from build123d import *

# Parameters (mm, degrees)
SKETCH1_W           = 80
SKETCH1_H           = 14
BOSS_EXTRUDE1_DEPTH = 2
SKETCH2_W           = 80
SKETCH2_H           = 7.4
SKETCH2_H_2         = 4.9
BOSS_EXTRUDE2_DEPTH = 2
SKETCH3_W           = 28.7
SKETCH3_H           = 7
BOSS_EXTRUDE3_DEPTH = 4
BOSS_EXTRUDE4_DEPTH = 80
CUT_EXTRUDE1_DEPTH  = 1
BOSS_EXTRUDE5_DEPTH = 1.8
SKETCH7_W           = 47.6
SKETCH7_H           = 7.55
CUT_EXTRUDE2_DEPTH  = 1


with BuildPart() as part:
    # Sketch1 → Boss-Extrude1 (new body)
    with BuildSketch(Plane(origin=(0, 0, 0), x_dir=(1, 0, 0), z_dir=(0, 1, 0))):
        with Locations((32.454545455, 2.136363636)):
            Rectangle(SKETCH1_W, SKETCH1_H)
    extrude(amount=BOSS_EXTRUDE1_DEPTH)

    # Sketch2 → Boss-Extrude2 (add)
    with BuildSketch(Plane(origin=(0, 2, 0), x_dir=(1, 0, 0), z_dir=(0, 1, 0))):
        with Locations((32.454545455, -1.163636364)):
            Rectangle(SKETCH2_W, SKETCH2_H)
        with Locations((32.454545455, 6.686363636)):
            Rectangle(SKETCH2_W, SKETCH2_H_2)
    extrude(amount=BOSS_EXTRUDE2_DEPTH)

    # Sketch3 → Boss-Extrude3 (add)
    with BuildSketch(Plane.XZ):
        with Locations((6.804545455, -12.636363636)):
            Rectangle(SKETCH3_W, SKETCH3_H)
    extrude(amount=-BOSS_EXTRUDE3_DEPTH)

    # Sketch4 → Boss-Extrude4 (add)
    with BuildSketch(Plane.ZY.offset(7.545454545)):
        Polygon((-2.536363636, 2), (-2.686363636, 4), (-2.536363636, 4), align=None)
        Polygon((-4.236363636, 2), (-4.236363636, 4), (-4.086363636, 4), align=None)
    extrude(amount=-BOSS_EXTRUDE4_DEPTH)

    # Sketch5 → Cut-Extrude1 (cut)
    with BuildSketch(Plane.XZ):
        Polygon((-7.545454545, 4.863636364), (72.454545455, 4.863636364), (72.454545455, -9.136363636), (21.154545455, -9.136363636), (21.154545455, -16.136363636), (-7.545454545, -16.136363636), align=None)
    extrude(amount=-CUT_EXTRUDE1_DEPTH, mode=Mode.SUBTRACT)

    # Sketch6 → Boss-Extrude5 (add)
    with BuildSketch(Plane.XZ.offset(-1)):
        Polygon((21.154545455, -9.136363636), (72.454545455, -9.136363636), (72.454545455, -11.136363636), (23.154545455, -11.136363636), (23.154545455, -16.136363636), (21.154545455, -16.136363636), (21.154545455, -11.136363636), align=None)
    extrude(amount=-BOSS_EXTRUDE5_DEPTH)

    # Sketch7 → Cut-Extrude2 (cut)
    with BuildSketch(Plane(origin=(0, 4, 0), x_dir=(1, 0, 0), z_dir=(0, 1, 0))):
        with Locations((45.254545455, -1.088636364)):
            Rectangle(SKETCH7_W, SKETCH7_H)
    extrude(amount=-CUT_EXTRUDE2_DEPTH, mode=Mode.SUBTRACT)


solid = part.part
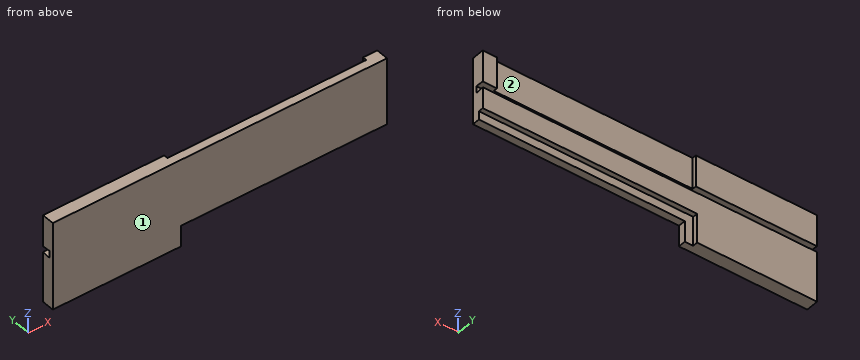
Source: CAD feature listing. Evaluate the final solid. Frame: model axes, mm. Face numbers are marked on the shaded views. Round coordinates to 2 decimals unless told otherwise and drop trailing zeros. Loops run counter-clockwise (first coordinate to the right, second up) from the corner with the lowest first, then second, coordinate; pieces in that order, holes last. Notation, with made-up numbers: M 7.25,36 L 32.25,36 A24 ccw 32.25,70 Z; hole C 89,-13 d11. An arc over 180 degrees is marked long. Answer as CSV lines item,"result".
Q1. Contact query for flat-ended pins moving along their axis: pin 1 (0.6 mm diameter, centred on x = 45, y = 3.5, fed in from -Z); pin 2 (3.5 mm diameter, centred on x = 42.5, z = 1, fed in from +Y); pin 3 (0.9 mm diameter, centred on x = 59, y = 1.5, fed in from -Z). Output: stop coordinate, or through.
Verdict:
pin 1,"stops at z = -9.14"
pin 2,"stops at y = 3"
pin 3,"stops at z = -11.14"
Q2. Cut plane A-A (x = 61). Return the cut outline in (y, z), plus the area to 3 significant figures.
Verdict:
outline,"M 1,-11.14 L 2.8,-11.14 L 2.8,-9.14 L 4,-9.14 L 4,-4.09 L 2,-4.24 L 2,-2.54 L 3,-2.61 L 3,4.86 L 1,4.86 Z"
area,"35.0 mm^2"
Q3. Cut plane D-D (x = 12.5). Return the cut outline in (y, z), plus the area to 3 significant figures.
Verdict:
outline,"M 1,-16.14 L 4,-16.14 L 4,-4.09 L 2,-4.24 L 2,-2.54 L 4,-2.69 L 4,4.86 L 1,4.86 Z"
area,"59.9 mm^2"
Q4. Cut plane C-C (z = -1.25). Return the cut outline in (x, y), plus the area to 3 significant figures.
Verdict:
outline,"M -7.55,1 L 72.45,1 L 72.45,4 L 69.05,4 L 69.05,3 L 21.45,3 L 21.45,4 L -7.55,4 Z"
area,"192 mm^2"
Q5. Line query: line 1 along Z through (x, y) = (20.5, 2.15); line 2 along X through (y, z) = (1.5, -14.25); line 3 along Y through (x, z) = (48.5, -3.25). Output: solid intervals per line, ascending.
Verdict:
line 1,"z = -16.14 to -4.23, -2.55 to 4.86"
line 2,"x = -7.55 to 23.15"
line 3,"y = 1 to 2"
Q6. Pull-direction query (X, two-part tool) for the marked faces 1 and 2; classes: +X half, -X half, draft (parallel to the pull), parting line (faces both ways), or undercut.
Verdict:
face 1,"draft"
face 2,"undercut"
Q7. Cut plane B-B (y = 3.5). Return the cut outline in (x, z), plus the area to 3 significant figures.
Verdict:
outline,"M -7.55,-16.14 L 21.15,-16.14 L 21.15,-9.14 L 72.45,-9.14 L 72.45,-4.12 L -7.55,-4.12 Z; M -7.55,-2.65 L 21.45,-2.65 L 21.45,4.86 L -7.55,4.86 Z; M 69.05,-2.65 L 72.45,-2.65 L 72.45,4.86 L 69.05,4.86 Z"
area,"845 mm^2"
